Geometry check sheet. Reference: the model listing, model coordinates, mm. Face numbers are marked on the shaded views. Give positions to 0.01 mm unless a question says otherwise; leave off trailing zeros. Loops run counter-clockwise (first coordinate to the right, second up) from the corner with the lowest first, then second, coordinate; pieces in that order, holes last. Notation, with made-up numbers: (23, 39) -> (50, 39) arc R34 cw to (50, 70) -> close; hole circle Ø4 at (72, 80.25). An arc over 180 degrees is marked (long way). Answer as a JSON object with one key per item and string values.
Autodesk Inventor part; units mm, degrees
ref_plane "YZ Plane" through (0, 0, 0) normal (1, 0, 0) x (0, 1, 0)
ref_plane "XZ Plane" through (0, 0, 0) normal (0, 1, 0) x (-1, 0, 0)
ref_plane "XY Plane" through (0, 0, 0) normal (0, 0, 1) x (1, 0, 0)
sketch "Sketch3" plane through (0, 0, 0) normal (0, 1, 0) x (-1, 0, 0)
  line L0 (55, 0) -> (0, 0)
  line L1 (0, 0) -> (0, -20)
  line L2 (0, -20) -> (55, -20)
  line L3 (55, -20) -> (55, 0)
  dimension "d9" = 55
  dimension "d10" = 20
extrude "Plate1" add sketch "Sketch3" along normal blind 2.032
sketch "Sketch4" plane through (-52.968, 0, 0) normal (-1, 0, 0) x (0, -1, 0)
  line L0 (0, -20) -> (0, 0)
  line L1 (0, 0) -> (-40, 0)
  line L2 (-40, 0) -> (-40, -20)
  line L3 (-40, -20) -> (0, -20)
edge flange "Flange1" height 40 angle 90 thickness 2.032 bend radius 2.032 thickness toward (-1, 0, 0) relief tear relief width 2.032 relief depth 1.016 corner gap 2.032 corner form 0 edges at (-55, 2.032, -10) (0, 2.032, -10) wall of the first edge with corners at (-52.968, 0, -20) (-52.968, 0, 0) (-52.968, 40, 0) (-52.968, 40, -20)
bend "Bend1"
corner "Corner1"
sketch "Sketch5" plane through (0, 40, 0) normal (1, 0, 0) x (0, 0, -1)
  line L0 (0, -35.936) -> (20, -35.936)
  line L1 (0, -35.936) -> (20, -35.936)
  line L2 (20, 0) -> (20, -35.936)
  line L3 (0, 0) -> (20, 0)
  line L4 (0, -35.936) -> (0, 0)
  line L5 (20, -35.936) -> (20, 0)
  line L6 (20, -17.968) -> (0, -17.968) construction
  line L7 (0, -35.936) -> (0, 0)
  point P0 (0, -40)
  point P1 (10, -5.468)
  point P2 (10, -17.968)
  point P3 (10, -30.468)
  point P4 (10, -35.936)
  point P5 (10, -17.968)
  dimension "d22" = 12.5
  dimension "d23" = 12.5
hole "Hole1" at (0, 9.532, -10) at (0, 34.532, -10) direction (-1, 0, 0) diameter 3.4 depth 55
hole "Hole2" at (0, 22.032, -10) direction (-1, 0, 0) diameter 14 depth 55
fillet "Fillet1" radius 6.7625 4 edges at (-53.984, 40, 0) (-53.984, 40, -20) (-1.016, 40, -20) (-1.016, 40, 0)
sketch "Sketch6" plane through (0, 2.032, 0) normal (0, 1, 0) x (1, 0, 0)
  line L0 (-4.064, 0) -> (-4.064, 20)
  line L1 (-50.936, 20) -> (-4.064, 20)
  line L2 (-50.936, 20) -> (-50.936, 0)
  line L3 (-4.064, 0) -> (-50.936, 0)
  line L4 (-4.064, 0) -> (-4.064, 20)
  line L5 (-4.064, 10) -> (-14.064, 10) construction
  line L6 (-40.936, 10) -> (-50.936, 10) construction
  point P0 (0, 0)
  dimension "d39" = 10
hole "Hole3" at (-40.936, 2.032, -10) at (-14.064, 2.032, -10) direction (0, -1, 0) diameter 3.4 end through all
sketch "Sketch7" plane through (-50.936, 0, 0) normal (0, 0, 1) x (1, 0, 0)
  line L0 (48.904, 4.064) -> (50.936, 4.064)
  arc A0 (46.872, 2.032) -> (48.904, 4.064) centre (46.872, 4.064) ccw
  line L1 (46.872, 0) -> (46.872, 2.032)
  arc A1 (46.872, 0) -> (50.936, 4.064) centre (46.872, 4.064) ccw
  line L2 (-4.064, 4.064) -> (-2.032, 4.064)
  arc A2 (-4.064, 4.064) -> (0, 0) centre (0, 4.064) ccw
  line L3 (0, 2.032) -> (0, 0)
  arc A3 (-2.032, 4.064) -> (0, 2.032) centre (0, 4.064) ccw
  arc A4 (-2.032, 4.064) -> (0, 2.032) centre (0, 4.064) ccw
  line L4 (-2.032, 4.064) -> (-2.032, 2.032)
  line L5 (-2.032, 2.032) -> (0, 2.032)
  arc A5 (-4.064, 4.064) -> (0, 0) centre (0, 4.064) ccw
  line L6 (0, 0) -> (-4.064, 0)
  line L7 (-2.032, 4.064) -> (-4.064, 4.064)
  line L8 (-4.064, 0) -> (-4.064, 4.064)
  arc A6 (46.872, 2.032) -> (48.904, 4.064) centre (46.872, 4.064) ccw
  line L9 (48.904, 4.064) -> (48.904, 2.032)
  line L10 (48.904, 2.032) -> (46.872, 2.032)
  line L11 (0, 0) -> (46.872, 0)
  line L12 (46.872, 0) -> (50.936, 0)
  line L13 (50.936, 0) -> (50.936, 4.064)
  point P0 (50.936, 0)
  point P1 (0, 0)
extrude "Extrusion3" cut sketch "Sketch7" against normal through all contours L9 L10 A0 | A3 L5 L4
extrude "Extrusion4" add sketch "Sketch7" against normal up to surface (20 mm away) contours L13 L12 A1 | A2 L6 L8
equation "\"d29\" = Thickness"
equation "\"d11\" = Thickness"
equation "\"d12\" = BendReliefWidth"
equation "\"d13\" = BendReliefDepth"
equation "\"d14\" = MinimumRemnant"
equation "\"d15\" = TransitionRadius"
equation "\"d18\" = BendRadius"
equation "\"d19\" = CornerReliefSize"
equation "\"d20\" = GapSize"
equation "\"d21\" = JacobiRadiusSize"
equation "\"BendRadius\" = Thickness"
equation "\"BendReliefWidth\" = Thickness"
equation "\"BendReliefDepth\" = 0.5 * Thickness"
equation "\"CornerReliefSize\" = 4 * Thickness"
equation "\"MinimumRemnant\" = 2 * Thickness"
equation "\"TransitionRadius\" = BendRadius"
equation "\"JacobiRadiusSize\" = BendRadius"
equation "\"GapSize\" = Thickness"
properties part number "Z Idle Mount-RP"
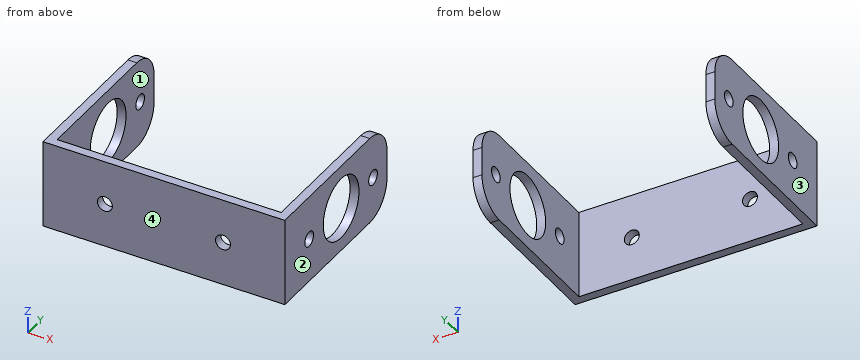
1) Section check C-C on x = -28. Record the cut outline in (y, z), plus the area to 3 significant figures.
Geometry check:
{"outline": "(0, -20) -> (2.03, -20) -> (2.03, 0) -> (0, 0) -> close", "area": "40.6 mm2"}
2) Section check B-B on y = 19. Record the cut outline in (x, z), plus the area to 3 significant figures.
Geometry check:
{"outline": "(-55, -20) -> (-52.97, -20) -> (-52.97, -16.31) -> (-55, -16.31) -> close; (-55, -3.69) -> (-52.97, -3.69) -> (-52.97, 0) -> (-55, 0) -> close; (-2.03, -20) -> (0, -20) -> (0, -16.31) -> (-2.03, -16.31) -> close; (-2.03, -3.69) -> (0, -3.69) -> (0, 0) -> (-2.03, 0) -> close", "area": "30.0 mm2"}
3) Section check D-D on z = -10. Count the separate pieces of the cut face and the enclosed holes in it, plus the area to 3 significant figures.
Geometry check:
{"separate pieces": "9", "enclosed holes": "0", "area": "168 mm2"}
4) Depth check by flat-ended pin: P1, Ø10, axis at x = -23, z = -11, coming from the +Y side; P2, Ø2, axis at x = -14.064, z = -10, coming from the -Y side. Enter the tip coordinate at first touch or a pass-through.
Geometry check:
{"P1": "stops at y = 2.03", "P2": "passes through"}
5) Section check A-A on y = 6. Record the cut outline in (x, z), plus the area to 3 significant figures.
Geometry check:
{"outline": "(-55, -20) -> (-52.97, -20) -> (-52.97, 0) -> (-55, 0) -> close; (-2.03, -20) -> (0, -20) -> (0, 0) -> (-2.03, 0) -> close", "area": "81.3 mm2"}
6) Draft check along X on the marked faces 1, 2, 3 and 4. Enter one of: pulls with the +X half, pulls with the -X half, needs draft (parallel to the pull), parting line crosses it, or undercut.
Geometry check:
{"face 1": "undercut", "face 2": "pulls with the +X half", "face 3": "pulls with the -X half", "face 4": "needs draft"}
7) Material ranges on line 1 along Y through (x, z) = (-1.4, -10); line 2 along X through (y, z) = (0.85, -10); line 3 along X through (y, z) = (13.5, -11), recorded low to high. Write a range as from..to.
Geometry check:
{"line 1": "y = 0..7.83, 11.23..15.03, 29.03..32.83, 36.23..40", "line 2": "x = -55..-42.64, -39.24..-15.76, -12.36..0", "line 3": "x = -55..-52.97, -2.03..0"}
